Could you check a few things on this drawing? It's one solid part, dimensions in mm from its lowest x, y, z. A direction names the side the tool comes from. Give positions to 0.01 mm unless a question says otherwise; leave off trailing zeros. Write each loop counter-clockwise with the first axis right and the second up, starting at its lowest first coordinate (ties: lowest second). Pieces come first, ordered by that corner, then holes. Notation, with made-up numbers: (61, 69) -> (77, 69) arc R19 cw to (77, 94) -> close; hole circle Ø5 at (74.25, -15). An arc over 180 degrees is marked (long way). Use CSV: the item, a comma, the result in double quotes. Start each with the question number.
(1) Suppose I cut it at A-A on z = 62.5. List the corners of the cut face in (x, y) for me.
(2) I need wall thicknesses on L1, parallel to Y at x = 14, z = 62; L2, parallel to Z at x = 30, y = 62 (3 decimals); L3, parallel to Z at x = 7, y = 62. Which ranges of each line are inside material? Lowest first, please. Write a range as [from, to].
(3) Suppose I cut it at C-C on x = 30. List the corners of the cut face in (y, z) for me, plus the area to 3 significant figures.
(4) Which directions (+Z, -Z, +X, -X, +Y, -Y) give clear straight access to the entire face, cutting with the end or side of a thin tool? Please do the marked faces 5 and 6.
(5) If we mould it in two halves opening along Z, with no side actions, what happens to the marked faces 1, 2, 3 and 4? For each: pulls with the +Z half, pulls with the -Z half, needs draft (parallel to the pull), parting line crosses it, or undercut.
(6) Suppose I cut it at B-B on x = 6.5. List the corners of the cut face in (y, z) for me.
(7) For pin 1 Ø4 at (x, z) = (20.5, 74.5) entering from +Y; pin 2 Ø2 at (x, y) = (23.5, 29) entering from +Z; pin 3 Ø1.8 at (x, y) = (17.5, 62.5) entering from -Z, each with a flat end and sliding along its axis, tell me the tip position at first contact or that it passes through.
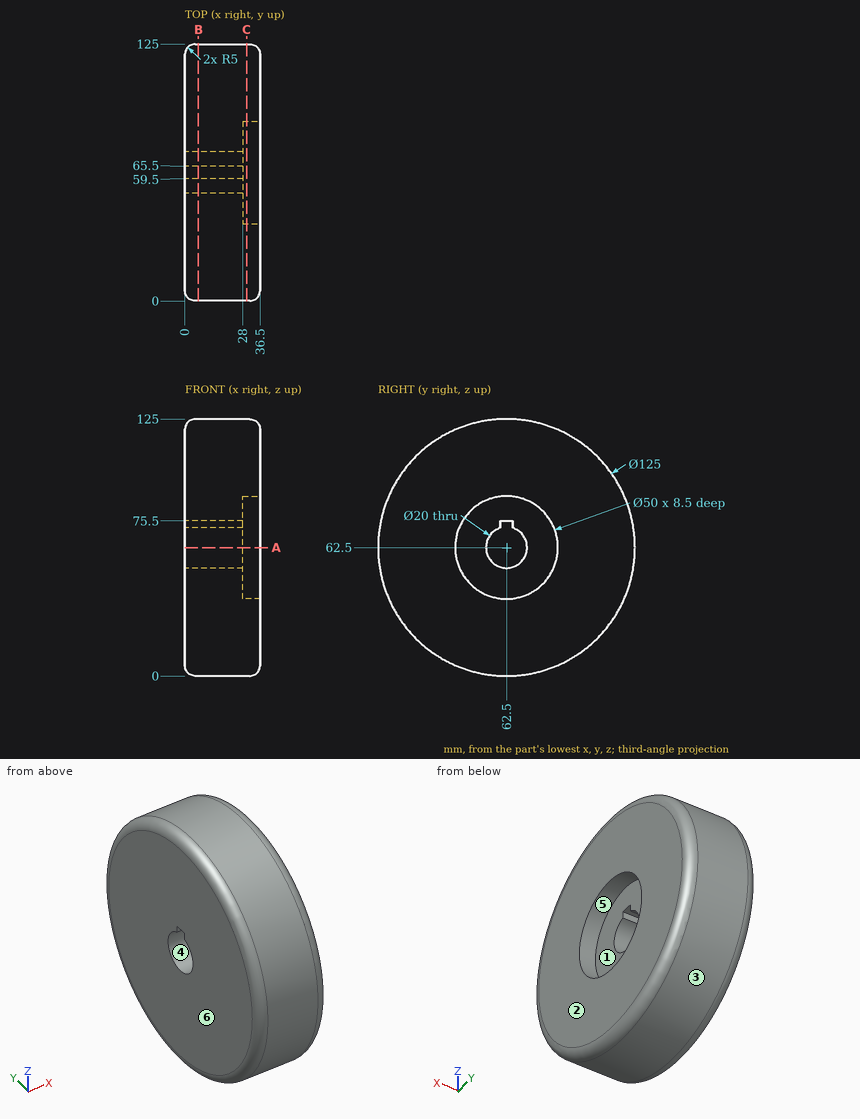
Geometry says:
1,outline,"(0, 5) arc R5 ccw to (5, 0) -> (31.5, 0) arc R5 ccw to (36.5, 5) -> (36.5, 37.5) -> (28, 37.5) -> (28, 52.5) -> (0, 52.5) -> close; (0, 72.5) -> (28, 72.5) -> (28, 87.5) -> (36.5, 87.5) -> (36.5, 120) arc R5 ccw to (31.5, 125) -> (5, 125) arc R5 ccw to (0, 120) -> close"
2,L1,"[0, 52.51], [72.49, 125]"
2,L2,"[0.002, 37.505], [87.495, 124.998]"
2,L3,"[0, 52.51], [75.5, 125]"
3,outline,"circle Ø125 at (62.5, 62.5); hole circle Ø50 at (62.5, 62.5)"
3,area,"10,300 mm²"
4,face 5,"+X"
4,face 6,"+Z, -Z, -X, +Y, -Y"
5,face 1,"undercut"
5,face 2,"needs draft"
5,face 3,"parting line crosses it"
5,face 4,"undercut"
6,outline,"circle Ø125 at (62.5, 62.5); hole (59.5, 72.04) arc R10 ccw (long way) to (65.5, 72.04) -> (65.5, 75.5) -> (59.5, 75.5) -> close"
7,pin 1,"y = 124.19"
7,pin 2,"z = 115.89"
7,pin 3,"z = 0"
